Verification items for this drawing (mm, ordinates from the low corner). Coordinates: 2 decimals unless noted, no trailing zeros. Order: outer loops, then holes, each group sorted by start corner. A loop starts at its lowest first (then second) coordinate and runs counter-clockwise, first axis right, second up. Notation, with made-up numbers: (61.25, -28.75) -> (93.25, -28.75) arc R22 cw to (93.25, -20.75) -> close; hole circle Ø5 at (81, 66). An arc over 180 degrees is marked (long way). Write each question's results on one line, items separated by ' | '. Start each with the question number.
(1) Thickness scan on probe 1 along Y at (x, z) = (20, 0.5); probe 2 along Z at (x, y) = (19.5, 18). Record the ranges inside material, lowest first. Write a range as [from, to].
(2) Cross-section at B-B on y = 13.5. Enter the section's corners in (x, z).
(3) Go/stop test with a flat-tipped pin: pin 1 (7.5 mm diameter, centred on x = 23, y = 13, fed in from -Z). Record where the tip stops, or that it passes through.
(4) Cross-section at C-C on x = 20. Enter the section's corners in (y, z), and give its area (3 significant figures).
(5) Draft check along X on the marked faces 1, 2, 3 and 4. Enter one of: +X half, -X half, draft (parallel to the pull), parting line (faces both ways), or undercut.
(6) Cross-section at A-A on z = 1.25. Enter the section's corners in (x, y), and give its area (3 significant figures).
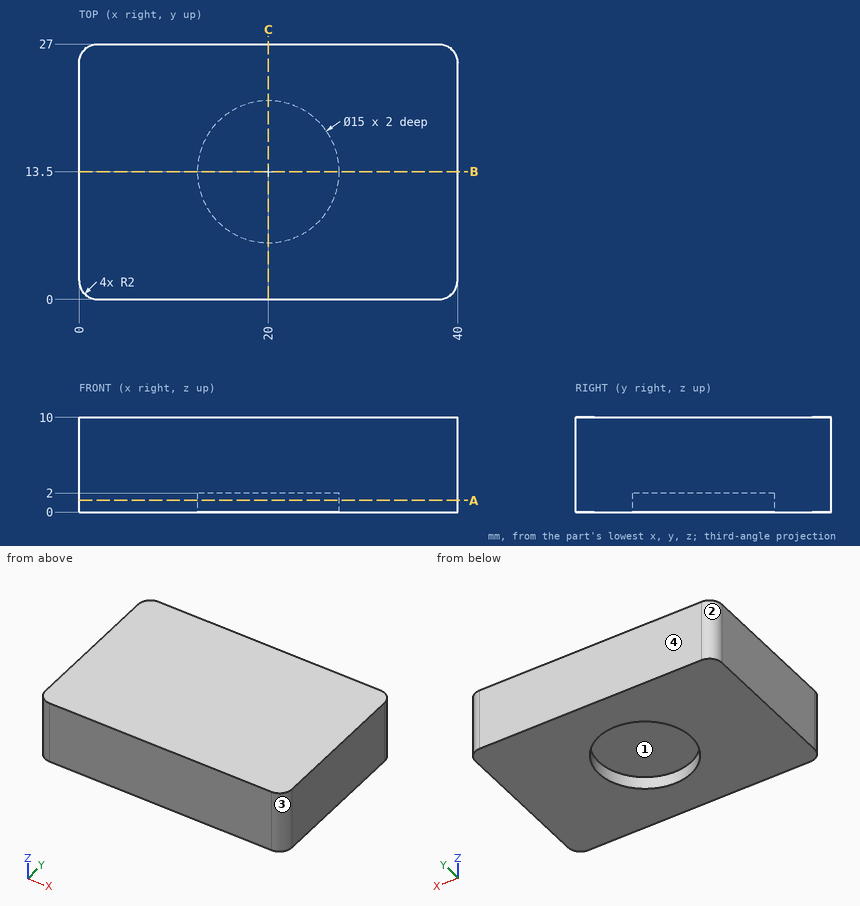
Results are:
1) probe 1: y = [0, 6], [21, 27] | probe 2: z = [2, 10]
2) outline: (0, 0) -> (12.5, 0) -> (12.5, 2) -> (27.5, 2) -> (27.5, 0) -> (40, 0) -> (40, 10) -> (0, 10) -> close
3) pin 1: stops at z = 2
4) outline: (0, 0) -> (6, 0) -> (6, 2) -> (21, 2) -> (21, 0) -> (27, 0) -> (27, 10) -> (0, 10) -> close | area: 240 mm2
5) face 1: undercut | face 2: -X half | face 3: +X half | face 4: draft
6) outline: (0, 2) arc R2 ccw to (2, 0) -> (38, 0) arc R2 ccw to (40, 2) -> (40, 25) arc R2 ccw to (38, 27) -> (2, 27) arc R2 ccw to (0, 25) -> close; hole circle Ø15 at (20, 13.5) | area: 900 mm2
